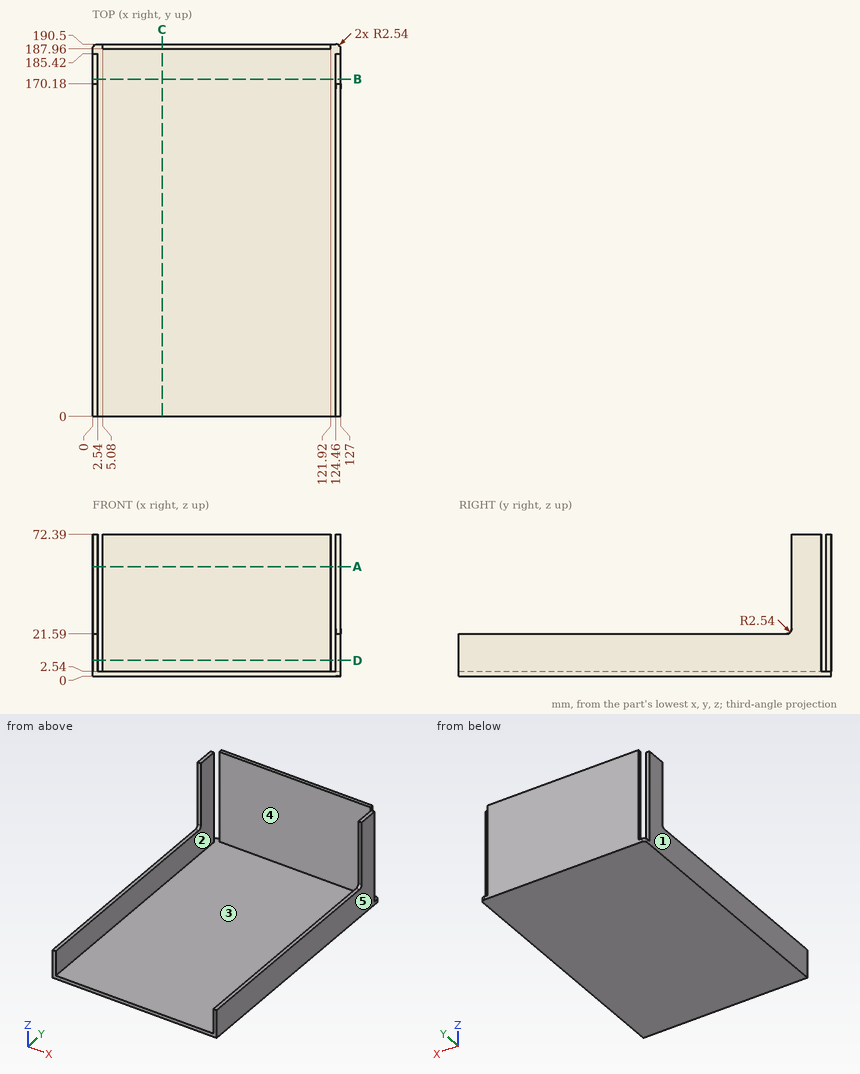
Check sheet for the drawn part. Datum: minimum x, y, z corner. Units: mm. A direction names the side the tool comes from. Give positions to 0.01 mm unless a question says otherwise; leave off trailing zeros. Order: outer loops, then holes, each group sorted by start corner. A loop starts at its lowest first (then second) coordinate and runs counter-clockwise, first axis right, second up. Notation, with made-up numbers: (55, 30.5) -> (71, 30.5) arc R22 cw to (71, 57.5) -> close; hole circle Ø8 at (-28, -36). An arc over 180 degrees is marked (long way). Use a Markdown table: item, result.
1) Section check C-C, the plane x = 35.5. Record the boundary of the cut face in (y, z), then the cut area to 3 significant figures.
Results:
| item | result |
|---|---|
| outline | (0, 0) -> (190.5, 0) -> (190.5, 72.39) -> (187.96, 72.39) -> (187.96, 2.54) -> (0, 2.54) -> close |
| area | 661 mm² |
2) Mould release check, pull along X, two halves, no side actions. Record for the marked faces 3, 4 and 5: pulls with the +X half, pulls with the -X half, needs draft (parallel to the pull), parting line crosses it, or undercut.
Results:
| item | result |
|---|---|
| face 3 | undercut |
| face 4 | needs draft |
| face 5 | pulls with the +X half |
3) Section check A-A, the plane z = 56. Record the boundary of the cut face in (x, y).
Results:
| item | result |
|---|---|
| outline | (0, 170.18) -> (2.54, 170.18) -> (2.54, 185.42) -> (0, 185.42) -> close; (5.08, 187.96) -> (121.92, 187.96) -> (121.92, 190.5) -> (5.08, 190.5) -> close; (124.46, 170.18) -> (127, 170.18) -> (127, 185.42) -> (124.46, 185.42) -> close |
4) Tool access check on the marked faces 1 and 2. Record the directions out of +Z, -Z, +X, -X, +Y, -Y that give a thin tool (end or side, any length) a straight path to the whole face; none if there is none.
Results:
| item | result |
|---|---|
| face 1 | +Z, -Z, -X, +Y, -Y |
| face 2 | +Z, +Y, -Y |
5) Section check B-B, the plane y = 172.5. Record the boundary of the cut face in (x, z), then the cut area to 3 significant figures.
Results:
| item | result |
|---|---|
| outline | (0, 0) -> (127, 0) -> (127, 72.39) -> (124.46, 72.39) -> (124.46, 2.54) -> (2.54, 2.54) -> (2.54, 72.39) -> (0, 72.39) -> close |
| area | 677 mm² |
6) Section check D-D, the plane z = 8. Record the boundary of the cut face in (x, y).
Results:
| item | result |
|---|---|
| outline | (0, 0) -> (2.54, 0) -> (2.54, 185.42) -> (0, 185.42) -> close; (5.08, 187.96) -> (121.92, 187.96) -> (121.92, 190.5) -> (5.08, 190.5) -> close; (124.46, 0) -> (127, 0) -> (127, 185.42) -> (124.46, 185.42) -> close |
7) Depth check by flat-ended pin: pin 1 Ø1.5 at (x, y) = (28.5, 29.5) entering from -Z; pin 2 Ø1.3 at (x, z) = (1.5, 43.5) entering from -Y; pin 3 Ø0.8 at (y, z) = (189, 31) entering from +X; pin 4 Ø1.3 at (x, y) = (125.5, 104.5) entering from +Z. Enter the tip coordinate at first touch or a pass-through.
Results:
| item | result |
|---|---|
| pin 1 | z = 0 |
| pin 2 | y = 170.18 |
| pin 3 | x = 121.92 |
| pin 4 | z = 21.59 |
8) Material ranges on probe 1 along X at (y, z) = (179, 60); probe 2 along Z at (x, y) = (29.5, 98); probe 3 along Y at (x, z) = (17, 42), recorded low to high.
Results:
| item | result |
|---|---|
| probe 1 | 0 to 2.54, 124.46 to 127 |
| probe 2 | 0 to 2.54 |
| probe 3 | 187.96 to 190.5 |
